Read the model definition and answer for the solid it produces. Units are mm, in the model's axes. A direction names the side the tool comes from. Give positions to 0.01 mm unless a question says otherwise; leave off trailing zeros. Write each loop counter-clockwise with the first axis right and the second up, starting at its lowest first coordinate (ties: lowest second). Pieces come first, ordered by that corner, then holes. Notation, with made-up numbers: M 58.25,-4.75 L 106.25,-4.75 A16 ccw 106.25,8.25 Z; hole C -11.75,-21 d2. An arc over 180 degrees is marked long. Put each result on its own line as item: value.
from build123d import *

# Parameters (mm, degrees)
SKETCH9_R           = 1.4986
BOSS_EXTRUDE2_DEPTH = 1
BOSS_EXTRUDE8_DEPTH = 1
BOSS_EXTRUDE3_DEPTH = 14
SKETCH12_W          = 63.348303519
SKETCH12_H          = 1.5
BOSS_EXTRUDE4_DEPTH = 14


with BuildPart() as part:
    # Sketch9 → Boss-Extrude2 (new body)
    with BuildSketch(Plane.XY):
        Polygon((0, 45.894331692), (15.488494665, 40.257085472), (21.11579715, 55.718259441), (31.638563481, 55.718259441), (42.161245631, 55.760350338), (47.850347546, 40.321809178), (63.316169409, 46.020964031), (63.494666021, 1.396989332), (62.229756161, 0.121919512), (31.75, 0), (1.27, 0), (0, 1.27), align=None)
        with Locations((60.94984, 2.54)):
            Circle(SKETCH9_R, mode=Mode.SUBTRACT)
        with Locations((21.082, 50.8)):
            Circle(SKETCH9_R, mode=Mode.SUBTRACT)
        with Locations((2.54, 41.91)):
            Circle(SKETCH9_R, mode=Mode.SUBTRACT)
        with Locations(Location((60.792126991, 42.026504254, 0), (0, 0, 180))):
            Circle(SKETCH9_R, mode=Mode.SUBTRACT)
        with Locations(Location((42.214715469, 50.842265431, 0), (0, 0, 180))):
            Circle(SKETCH9_R, mode=Mode.SUBTRACT)
        with Locations((2.45872, 20.32)):
            Circle(SKETCH9_R, mode=Mode.SUBTRACT)
    extrude(amount=BOSS_EXTRUDE2_DEPTH)

    # Sketch13 → Boss-Extrude8 (add)
    with BuildSketch(Plane(origin=(0, 0, 0), x_dir=(-1, 0, 0), z_dir=(0, 0, -1))):
        Polygon((-21.11579715, 55.718259441), (-23.047346454, 61.025246209), (-7.480797331, 66.691011442), (-55.947053109, 66.787943953), (-40.208483916, 61.059568484), (-42.161245631, 55.760350338), (-27.798035754, 50.098344964), align=None)
    extrude(amount=-BOSS_EXTRUDE8_DEPTH)

    # Sketch11 → Boss-Extrude3 (add)
    with BuildSketch(Plane.XY.offset(1)):
        Polygon((32.438774093, 58.231623033), (32.438774093, 9.039988), (63.464093904, 9.039988), (63.47009388, 7.54), (32.438774093, 7.54), (32.438774093, 1.27), (0, 1.27), (0, 2.77), (30.940876447, 2.77), (30.940876447, 58.152233865), (11.329502605, 65.290196119), (11.842533196, 66.699734913), (31.580765387, 59.515599958), (51.537117344, 66.779124082), (52.050147935, 65.369585287), align=None)
    extrude(amount=BOSS_EXTRUDE3_DEPTH)

    # Sketch12 → Boss-Extrude4 (add)
    with BuildSketch(Plane.XY.offset(1)):
        with Locations((31.67415176, 37.237468453)):
            Rectangle(SKETCH12_W, SKETCH12_H)
    extrude(amount=BOSS_EXTRUDE4_DEPTH)


solid = part.part
(1) Section B-B on y = 20.32 is taken. Determine the outline of the cut face in (x, z).
Result:
outline: M 0,0 L 0.96,0 L 0.96,1 L 0,1 Z; M 3.96,0 L 63.42,0 L 63.42,1 L 32.44,1 L 32.44,15 L 30.94,15 L 30.94,1 L 3.96,1 Z
(2) For a pull along Y with two mould halves and no side action, classify faces 1 (the face through (51.79, 66.08, 7.9)), 2 (the face through (16, 20, 1)), 3 (the face through (32, 32, 15)) as +Y half, -Y half, draft (parallel to the pull), parting line (faces both ways), or undercut.
Result:
face 1: +Y half
face 2: undercut
face 3: draft
(3) Section D-D on x = 2.54 is taken. Determine the outline of the cut face in (y, z), and give its area (3 significant figures).
Result:
outline: M 0,0 L 18.82,0 L 18.82,1 L 2.77,1 L 2.77,15 L 1.27,15 L 1.27,1 L 0,1 Z; M 21.82,0 L 40.41,0 L 40.41,1 L 37.99,1 L 37.99,15 L 36.49,15 L 36.49,1 L 21.82,1 Z; M 43.41,0 L 44.97,0 L 44.97,1 L 43.41,1 Z
area: 81.0 mm²
(4) Which of the six approach directions +Z, -Z, +X, -X, +Y, -Y give full straight-line access (tool end or side, diameter ignored) to faces 4 (the face through (11.582, 65.985, 7.902)), 5 (the face through (30.941, 19, 8)), 6 (the face through (48, 37.987, 8))?
Result:
face 4: +Z, -X, +Y
face 5: +Z, -X
face 6: +Z, +X
(5) Given pin 1 Ø2 at (x, y) = (23, 27) entering from +Z; pin 2 Ø1.5 at (x, z) = (37, 9.5) entering from -Y; pin 3 Ø5 at (y, z) = (41.5, 10.5) entering from -X, each flat-ended and moving along its own axis, determine where each tip first touches the part or whether it passes through.
Result:
pin 1: stops at z = 1
pin 2: stops at y = 7.54
pin 3: stops at x = 30.94
(6) Section C-C on z = 2 is taken. Determine the outline of the cut face in (x, y), and give its area (3 significant figures).
Result:
outline: M 0,1.27 L 32.44,1.27 L 32.44,7.54 L 63.47,7.54 L 63.46,9.04 L 32.44,9.04 L 32.44,36.49 L 63.35,36.49 L 63.35,37.99 L 32.44,37.99 L 32.44,58.23 L 52.05,65.37 L 51.54,66.78 L 31.58,59.52 L 11.84,66.7 L 11.33,65.29 L 30.94,58.15 L 30.94,37.99 L 0,37.99 L 0,36.49 L 30.94,36.49 L 30.94,2.77 L 0,2.77 Z
area: 335 mm²
(7) Straight lines are drawn through the part: line 1 along Y through (x, z) = (54, 8); line 2 along Y through (x, z) = (29.5, 7); line 3 along Y through (x, z) = (2.54, 0.75). For each, find the intervals that lie inside material, in ascending order. Write a range as from..to.
Result:
line 1: y = 7.54..9.04, 36.49..37.99
line 2: y = 1.27..2.77, 36.49..37.99, 58.68..60.27
line 3: y = 0..18.82, 21.82..40.41, 43.41..44.97
(8) Section A-A on x = 46 is taken. Determine the outline of the cut face in (y, z).
Result:
outline: M 0.06,0 L 45.34,0 L 45.34,1 L 37.99,1 L 37.99,15 L 36.49,15 L 36.49,1 L 9.04,1 L 9.04,15 L 7.54,15 L 7.54,1 L 0.06,1 Z; M 63.17,0 L 66.77,0 L 66.77,1 L 64.76,1 L 64.76,15 L 63.17,15 Z
